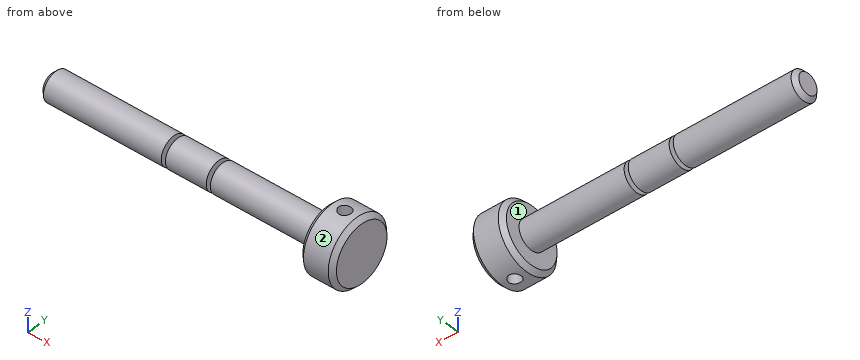
```python
from build123d import *

# Parameters (mm, degrees)
CHAMFER1_SIZE           = 2
CHAMFER2_SIZE           = 2.1213
SKETCH3_R               = 3
CUT_EXTRUDE1_DEPTH      = 135
CUT_EXTRUDE1_DEPTH_BACK = 135


with BuildPart() as part:
    # Sketch2 → Revolve1 (revolve)
    with BuildSketch(Plane.XY):
        Polygon((-76.638954869, 0), (74.714964371, 0), (74.714964371, 16), (58.361045131, 16), (58.361045131, 7), (6.961045131, 7), (6.961045131, 2.991686461), (4.961045131, 2.991686461), (4.961045131, 7), (-15.038954869, 7), (-15.038954869, 2.991686461), (-17.038954869, 2.991686461), (-17.038954869, 7), (-76.638954869, 7), align=None)
    revolve(axis=Axis((-76.638954869, 0, 0), (1, 0, 0)))

    # Chamfer1
    chamfer1_edges = [part.edges().sort_by_distance(p)[0] for p in [
        (-76.638954869, -7, 0),
    ]]
    chamfer(chamfer1_edges, length=CHAMFER1_SIZE)

    # Chamfer2
    chamfer2_edges = [part.edges().sort_by_distance(p)[0] for p in [
        (58.361045131, -16, 0),
        (74.714964371, -16, 0),
    ]]
    chamfer(chamfer2_edges, length=CHAMFER2_SIZE)

    # Sketch3 → Cut-Extrude1 (cut, two sides)
    with BuildSketch(Plane.XY) as cut_extrude1_sk:
        with Locations((66.538004751, 0)):
            Circle(SKETCH3_R)
    extrude(amount=CUT_EXTRUDE1_DEPTH, mode=Mode.SUBTRACT)
    extrude(cut_extrude1_sk.sketch, amount=-CUT_EXTRUDE1_DEPTH_BACK, mode=Mode.SUBTRACT)


solid = part.part
```
Here's how the part is built. I have some questions about the finished solid (model axes, mm). Face numbers are marked on the shaded views. A direction names the side the tool comes from. Coordinates: 2 decimals unless noted, no trailing zeros. Loops run counter-clockwise (first coordinate to the right, second up) from the corner with the lowest first, then second, coordinate; pieces in that order, holes last. Notation, with made-up numbers: M -13,11.5 L 33,11.5 A18 cw 33,45.5 Z; hole C 14.25,22.5 d5. An arc over 180 degrees is marked long. One line per item, written item: value.
1. On a 3-axis mill with a long thin cutter (end or side, diameter ignored), from which of +Z, -Z, +X, -X, +Y, -Y can I reach the whole of each face in a straight line? I mean the marked faces 1 and 2. Say none if no direction works.
Geometry says:
face 1: -X
face 2: +X, -X
2. Imagine slicing it at B-B (x = -36). List the corners of the cut face in (y, z) for me, and give its area (3 significant figures).
Geometry says:
outline: C 0,0 d14
area: 154 mm2
3. Please list where these lines run through material, in increasing order: probe 1 along X at (y, z) = (2.5, -5.5); probe 2 along X at (y, z) = (0, -12.5); probe 3 along X at (y, z) = (0, 6).
Geometry says:
probe 1: x = -75.6 to -17.04, -15.04 to 4.96, 6.96 to 64.88, 68.2 to 74.71
probe 2: x = 58.36 to 63.54, 69.54 to 74.71
probe 3: x = -75.64 to -17.04, -15.04 to 4.96, 6.96 to 63.54, 69.54 to 74.71
4. Will these pins go through, and if not, where does the flat tip stop? pin 1 Ø12 at (x, y) = (-15.5, -11.5) entering from +Z; pin 2 Ø4 at (x, z) = (-24, 3) entering from +Y; pin 3 Ø4 at (x, z) = (19.5, 2.5) entering from -Y.
Geometry says:
pin 1: stops at z = 4.31
pin 2: stops at y = 6.93
pin 3: stops at y = -6.98
